CAD build for the part. Positions are in the model's coordinates, mm. Face numbers are marked on the shaded views. Round coordinates to 2 decimals unless told otherwise and drop trailing zeros. Loops run counter-clockwise (first coordinate to the right, second up) from the corner with the lowest first, then second, coordinate; pieces in that order, holes last. Notation, with made-up numbers: (83, 27.25) -> (102, 27.25) arc R23 ccw to (102, 57.25) -> close; hole circle Ø3 at (36, 72). An arc over 180 degrees is marked (long way). Answer as CSV lines item,"result".
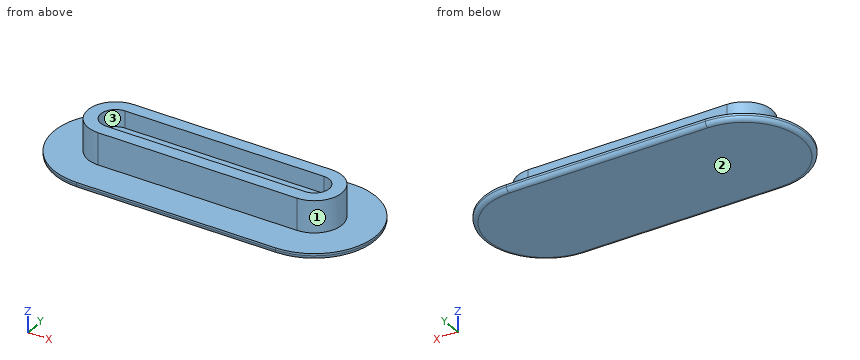
```python
from build123d import *

# Parameters (mm, degrees)
F0_W     = 47
F0_H     = 29
F1_DEPTH = 1.5
F2_W     = 47
F2_H     = 13
F3_DEPTH = 9
F4_T     = -3
F5_R     = 1
F6_DEPTH = 2


with BuildPart() as f1:
    # F0 (on Top) → F1 (new body)
    with BuildSketch(Plane.XY):
        Rectangle(F0_W, F0_H)
        with BuildLine():
            Line((23.5, 14.5), (23.5, -14.5))
            ThreePointArc((23.5, -14.5), (38, 0), (23.5, 14.5))
        make_face()
        with BuildLine():
            ThreePointArc((-23.5, 14.5), (-38, 0), (-23.5, -14.5))
            Line((-23.5, -14.5), (-23.5, 14.5))
        make_face()
    extrude(amount=F1_DEPTH)

    # F2 (on face) → F3 (join)
    with BuildSketch(Plane.XY):
        Rectangle(F2_W, F2_H)
        with BuildLine():
            Line((23.5, 6.5), (23.5, -6.5))
            ThreePointArc((23.5, -6.5), (30, 0), (23.5, 6.5))
        make_face()
        with BuildLine():
            ThreePointArc((-23.5, 6.5), (-30, 0), (-23.5, -6.5))
            Line((-23.5, -6.5), (-23.5, 6.5))
        make_face()
    extrude(amount=F3_DEPTH)

    # F4
    f4_openings = [f1.faces().sort_by_distance(p)[0] for p in [
        (0, 0, 9),
    ]]
    offset(amount=F4_T, openings=f4_openings)

    # F5
    f5_edges = [f1.edges().sort_by_distance(p)[0] for p in [
        (38, 0, 0),
        (0, -14.5, 0),
        (-38, 0, 0),
        (0, 14.5, 0),
    ]]
    fillet(f5_edges, radius=F5_R)

    # F6 (add): a face of the model
    f6_faces = [f1.faces().sort_by_distance(p)[0] for p in [
        (0, 0, 3),
    ]]
    extrude(f6_faces, amount=F6_DEPTH)


solid = f1.part
```
Q1. Slice it at B-B, the plane y = 0. Give the cut face in (x, z), and give its area (3 significant figures).
Results:
outline,"(-38, 1) arc R1 ccw to (-37, 0) -> (37, 0) arc R1 ccw to (38, 1) -> (38, 1.5) -> (30, 1.5) -> (30, 9) -> (27, 9) -> (27, 5) -> (-27, 5) -> (-27, 9) -> (-30, 9) -> (-30, 1.5) -> (-38, 1.5) -> close"
area,"348 mm2"
Q2. Slice it at A-A, the plane x = 21.5. Give the cut face in (y, z), and give its area (3 significant figures).
Results:
outline,"(-14.5, 1) arc R1 ccw to (-13.5, 0) -> (13.5, 0) arc R1 ccw to (14.5, 1) -> (14.5, 1.5) -> (6.5, 1.5) -> (6.5, 9) -> (3.5, 9) -> (3.5, 5) -> (-3.5, 5) -> (-3.5, 9) -> (-6.5, 9) -> (-6.5, 1.5) -> (-14.5, 1.5) -> close"
area,"113 mm2"
Q3. Probe L1, parallel to Y at x = 12.5, z = 8.75; L2, parallel to Z at x = -24.5, y = -11.5; L3, parallel to Y at x = 20, z = 2. List the from-to ranges inside material, lowest first. Write a range as [from, to].
Results:
L1,"[-6.5, -3.5], [3.5, 6.5]"
L2,"[0, 1.5]"
L3,"[-6.5, 6.5]"
Q4. Drop flat-ended pins along their axis: pin 1 Ø4 at (y, z) = (-3.5, 1) entering from -X; pin 2 Ø1.2 at (x, z) = (7, 8) entering from -Y; pin 3 Ø1.5 at (x, z) = (-26.5, 2) entering from -Y. Give the stop position or say it passes through.
Results:
pin 1,"x = -37.92"
pin 2,"y = -6.5"
pin 3,"y = -14.29"
Q5. Two-plate mould, pull along X, no slides. Class the marked faces 1, 2 and 3: pulls with the +X half, pulls with the -X half, needs draft (parallel to the pull), parting line crosses it, or undercut.
Results:
face 1,"pulls with the +X half"
face 2,"needs draft"
face 3,"undercut"
Q6. Slice it at C-C, the plane z = 3.75. Give the cut face in (x, y), and give its area (3 significant figures).
Results:
outline,"(-23.5, -6.5) -> (23.5, -6.5) arc R6.5 ccw to (23.5, 6.5) -> (-23.5, 6.5) arc R6.5 ccw to start"
area,"744 mm2"
